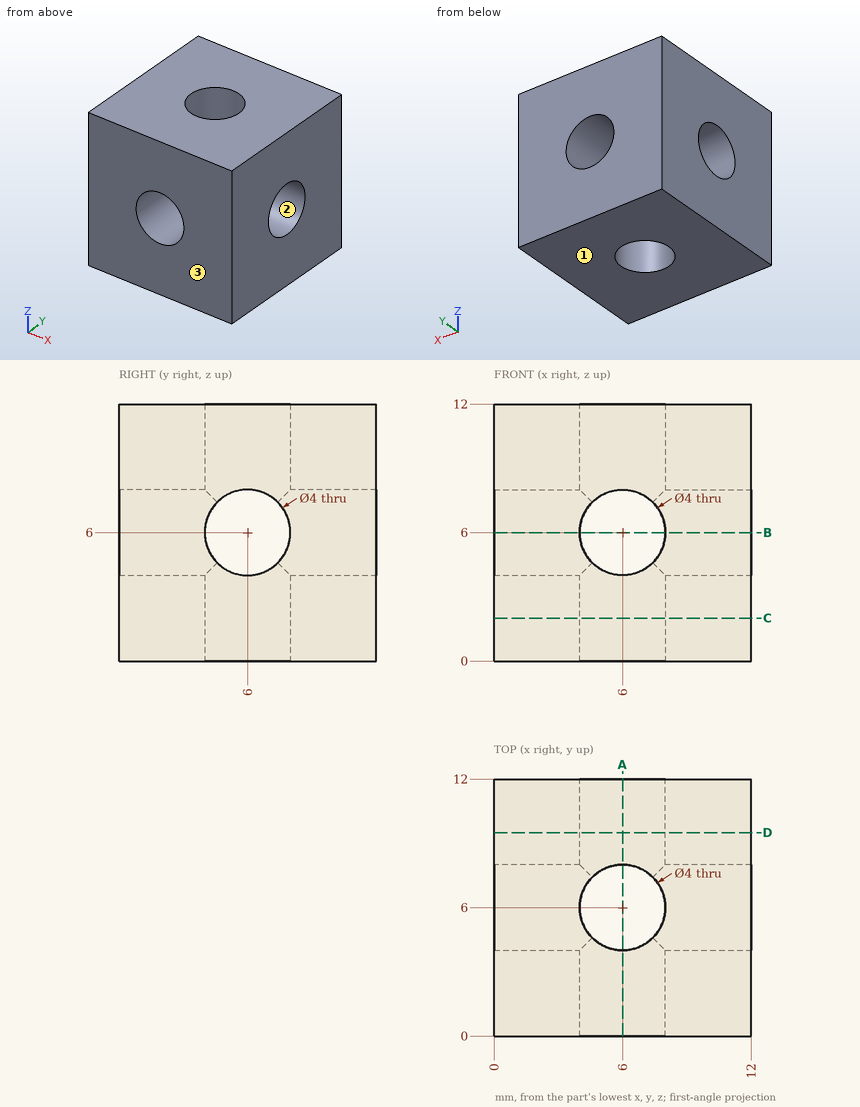
Source: three-view drawing plus pictorial views. Frame: mm from the lowest corner of the part. Round coordinates to 2 decimals unless told otherwise and drop trailing zeros. Order: outer loops, then holes, each group sorted by start corner. A loop starts at its lowest first (then second) coordinate and runs counter-clockwise, first axis right, second up. Notation, with made-up numbers: (-2, 82.25) -> (48, 82.25) arc R13 cw to (48, 90.25) -> close; hole circle Ø3 at (64.25, 23). An arc over 180 degrees is marked (long way). Use one line per item in the form item = value. Start each with the question number.
1. Line query: probe 1 along X at (y, z) = (11.25, 6). Output: solid intervals per line, ascending.
2. Draft query along Y for the marked faces 1, 2 and 3. Return one class per face: pulls with the +Y half, pulls with the -Y half, needs draft (parallel to the pull), parting line crosses it, or undercut.
3. Cut plane A-A (x = 6). Return the cut outline in (y, z).
4. Cut plane C-C (z = 2). Return the cut outline in (x, y), then the cut area to 3 significant figures.
Solution:
q1.probe_1 = 0 to 4, 8 to 12
q2.face_1 = needs draft
q2.face_2 = undercut
q2.face_3 = pulls with the -Y half
q3.outline = (0, 0) -> (4, 0) -> (4, 4) -> (0, 4) -> close; (0, 8) -> (4, 8) -> (4, 12) -> (0, 12) -> close; (8, 0) -> (12, 0) -> (12, 4) -> (8, 4) -> close; (8, 8) -> (12, 8) -> (12, 12) -> (8, 12) -> close
q4.outline = (0, 0) -> (12, 0) -> (12, 12) -> (0, 12) -> close; hole circle Ø4 at (6, 6)
q4.area = 131 mm^2
